Geometry: final body of the model. Coordinates: model frame, mm. Face numbers are marked on the shaded views. Give positions to 0.01 mm unless a question says otherwise; leave off trailing zeros. Loops run counter-clockwise (first coordinate to the right, second up) from the corner with the lowest first, then second, coordinate; pieces in that order, holes last.
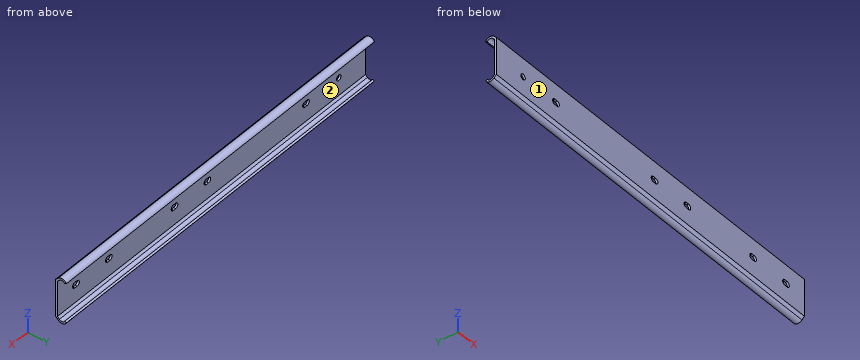
Autodesk Inventor part; units mm, degrees
ref_plane "IP0_XY" through (0, 0, 0) normal (-1, 0, 0) x (0, 0, -1)
ref_plane "IP0_YZ" through (0, 0, 0) normal (0, 0, -1) x (0, -1, 0)
ref_plane "IP0_ZX" through (0, 0, 0) normal (0, -1, 0) x (-1, 0, 0)
sketch "Esquisse_1" plane through (0, 0, 0) normal (1, 0, 0) x (0, 1, 0)
  arc A0 (8.5002, 15.4448) -> (1.9449, 16.4446) centre (4.8548, 13.5338) ccw
  line L0 (1.9449, 16.4446) -> (0, 14.5)
  line L1 (0, 14.5) -> (0, -14.5)
  line L2 (0, -14.5) -> (1.9449, -16.4446)
  arc A1 (1.9449, -16.4446) -> (8.5001, -15.4451) centre (4.8548, -13.5338) ccw
  line L3 (8.5001, -15.4451) -> (7.1713, -14.7492)
  arc A2 (3.0052, -15.3838) -> (7.1713, -14.7492) centre (4.8548, -13.5337) ccw
  line L4 (3.0052, -15.3838) -> (1.5, -13.879)
  line L5 (1.5, -13.879) -> (1.5, 13.879)
  line L6 (1.5, 13.879) -> (3.0052, 15.3838)
  arc A3 (7.1713, 14.7492) -> (3.0052, 15.3838) centre (4.8548, 13.5337) ccw
  line L7 (7.1713, 14.7492) -> (8.5002, 15.4448)
extrude "Extrusion1" add sketch "Esquisse_1" along normal blind 300
sketch "Sketch2" plane through (0, 0, -14.5) normal (0, -1, 0) x (1, 0, 0)
  point P0 (26, 14.5)
hole "Drilling 1" at (26, 0, 0) direction (0, 1, 0) diameter 4.3 depth 1.5
sketch "Esquisse_3" plane through (0, 0, 0) normal (0, 1, 0) x (-1, 0, 0)
  arc A0 (-56.9, -2.15) -> (-56.9, 2.15) centre (-56.9, 0) ccw
  line L0 (-56.9, 2.15) -> (-59.1, 2.15)
  arc A1 (-59.1, 2.15) -> (-59.1, -2.15) centre (-59.1, 0) ccw
  line L1 (-59.1, -2.15) -> (-56.9, -2.15)
extrude "Extrusion2" cut sketch "Esquisse_3" along normal blind 1.5
sketch "Esquisse_4" plane through (0, 0, 0) normal (0, 1, 0) x (-1, 0, 0)
  arc A0 (-152.9, -2.15) -> (-152.9, 2.15) centre (-152.9, 0) ccw
  line L0 (-152.9, 2.15) -> (-155.1, 2.15)
  arc A1 (-155.1, 2.15) -> (-155.1, -2.15) centre (-155.1, 0) ccw
  line L1 (-155.1, -2.15) -> (-152.9, -2.15)
extrude "Extrusion3" cut sketch "Esquisse_4" along normal blind 1.5
sketch "Esquisse_5" plane through (0, 0, 0) normal (0, 1, 0) x (-1, 0, 0)
  arc A0 (-184.9, -2.15) -> (-184.9, 2.15) centre (-184.9, 0) ccw
  line L0 (-184.9, 2.15) -> (-187.1, 2.15)
  arc A1 (-187.1, 2.15) -> (-187.1, -2.15) centre (-187.1, 0) ccw
  line L1 (-187.1, -2.15) -> (-184.9, -2.15)
extrude "Extrusion4" cut sketch "Esquisse_5" along normal blind 1.5
sketch "Esquisse_6" plane through (0, 0, 0) normal (0, 1, 0) x (-1, 0, 0)
  arc A0 (-248.9, -2.15) -> (-248.9, 2.15) centre (-248.9, 0) ccw
  line L0 (-248.9, 2.15) -> (-251.1, 2.15)
  arc A1 (-251.1, 2.15) -> (-251.1, -2.15) centre (-251.1, 0) ccw
  line L1 (-251.1, -2.15) -> (-248.9, -2.15)
extrude "Extrusion5" cut sketch "Esquisse_6" along normal blind 1.5
sketch "Esquisse_7" plane through (0, 0, 0) normal (0, 1, 0) x (-1, 0, 0)
  arc A0 (-280.9, -2.15) -> (-280.9, 2.15) centre (-280.9, 0) ccw
  line L0 (-280.9, 2.15) -> (-283.1, 2.15)
  arc A1 (-283.1, 2.15) -> (-283.1, -2.15) centre (-283.1, 0) ccw
  line L1 (-283.1, -2.15) -> (-280.9, -2.15)
extrude "Extrusion6" cut sketch "Esquisse_7" along normal blind 1.5
ref_plane "IP0_XY" through (0, 0, 0) normal (-1, 0, 0) x (0, 0, -1)
ref_plane "IP0_YZ" through (0, 0, 0) normal (0, 0, -1) x (0, -1, 0)
ref_plane "IP0_ZX" through (0, 0, 0) normal (0, -1, 0) x (-1, 0, 0)
ref_plane "IP1_XY" through (2.5, 0, 0) normal (1, 0, 0) x (0, 0, -1)
ref_plane "IP1_YZ" through (2.5, 0, 0) normal (0, 0, -1) x (0, 1, 0)
ref_plane "IP1_ZX" through (2.5, 0, 0) normal (0, 1, 0) x (1, 0, 0)
properties part number "MICHAUD CHAILLY B3 - 21 - 30 - 1"
Q1. Section query B-B, the plane y = 5.5. Return loops of the section in (x, z), and give its area (3 significant figures).
Q2. Section query A-A, the plane x = 202. Return loops of the section in (y, z), and give its area (3 significant figures).
Q3. Material intervals for probe 1 along Z at (x, y) = (26, 0.95); probe 2 along Z at (x, y) = (26, 1); probe 3 along Y at (x, z) = (88, 12), sorted ascending.
Q4. Mould query, pull axis Z, two halves, no side actions, for the marked faces 1 and 2. Classes: +Z half, -Z half, draft (parallel to the pull), parting line (faces both ways), or undercut.
Q5. Pin query (flat end, axial travel): pin 1 Ø14 at (x, z) = (96.5, 5) entering from +Y; pin 2 Ø0.8 at (x, y) = (250, 1) entering from -Z; pin 3 Ø5 at (x, y) = (259.5, 7) entering from -Z; pin 4 Ø1.6 at (x, y) = (250.5, 0.5) entering from +Z. Return the tip coordinate at first contact, or that it passes through.
Resolved:
1. outline: (0, -17.6) - (300, -17.6) - (300, -16.07) - (0, -16.07) - close; (0, 16.07) - (300, 16.07) - (300, 17.6) - (0, 17.6) - close
1. area: 918 mm2
2. outline: (0, -14.5) - (1.94, -16.44) arc R4.12 ccw to (8.5, -15.45) - (7.17, -14.75) arc R2.62 cw to (3.01, -15.38) - (1.5, -13.88) - (1.5, 13.88) - (3.01, 15.38) arc R2.62 cw to (7.17, 14.75) - (8.5, 15.44) arc R4.12 ccw to (1.94, 16.44) - (0, 14.5) - close
2. area: 68.8 mm2
3. probe 1: z = -15.45 to -2.15, 2.15 to 15.45
3. probe 2: z = -15.5 to -2.15, 2.15 to 15.5
3. probe 3: y = 0 to 1.5
4. face 1: draft
4. face 2: undercut
5. pin 1: stops at y = 1.5
5. pin 2: stops at z = -15.9
5. pin 3: stops at z = -17.65
5. pin 4: stops at z = 15.8
